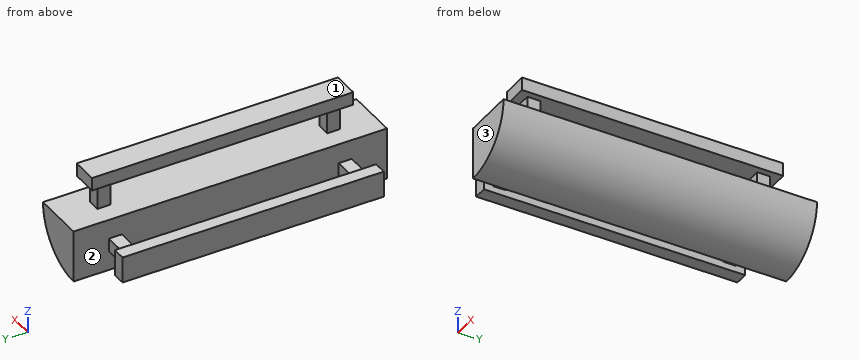
from build123d import *

# Parameters (mm, degrees)
SKETCH1_W               = 38.1
SKETCH1_H               = 101.6
BOSS_EXTRUDE1_DEPTH     = 304.8
CUT_EXTRUDE2_DEPTH      = 324.538575753
SKETCH3_W               = 12.7
SKETCH3_H               = 25.4
CUT_EXTRUDE3_DEPTH      = 324.538575753
CUT_EXTRUDE4_DEPTH      = 324.538575753
CUT_EXTRUDE5_DEPTH      = 152.4
SKETCH6_W               = 6.35
SKETCH6_H               = 6.35
BOSS_EXTRUDE2_DEPTH     = 12.7
SKETCH7_W               = 12.7
SKETCH7_H               = 127
BOSS_EXTRUDE3_DEPTH     = 6.35
MIRROR2_COPY_1_SKETCH_W = 6.35
MIRROR2_COPY_1_SKETCH_H = 6.35
MIRROR2_COPY_1_DEPTH    = 12.7


with BuildPart() as part:
    # Sketch1 → Boss-Extrude1 (new body)
    with BuildSketch(Plane(origin=(0, 0, 0), x_dir=(1, 0, 0), z_dir=(0, 1, 0))):
        with Locations((19.05, 50.8)):
            Rectangle(SKETCH1_W, SKETCH1_H)
    extrude(amount=BOSS_EXTRUDE1_DEPTH)

    # Sketch2 → Cut-Extrude2 (cut, through all)
    with BuildSketch(Plane.XZ):
        Polygon((12.7, -76.2), (38.1, -76.2), (38.1, 0), (0, 0), (0, -76.2), align=None)
    extrude(amount=-CUT_EXTRUDE2_DEPTH, mode=Mode.SUBTRACT)

    # Sketch3 → Cut-Extrude3 (cut, through all)
    with BuildSketch(Plane.XZ):
        with Locations((6.35, -88.9)):
            Rectangle(SKETCH3_W, SKETCH3_H)
    extrude(amount=-CUT_EXTRUDE3_DEPTH, mode=Mode.SUBTRACT)

    # Sketch4 → Cut-Extrude4 (cut, through all)
    with BuildSketch(Plane.XZ):
        with BuildLine():
            ThreePointArc((12.7, -101.6), (30.660512242, -94.160512242), (38.1, -76.2))
            Line((38.1, -76.2), (38.1, -101.6))
            Line((38.1, -101.6), (12.7, -101.6))
        make_face()
    extrude(amount=-CUT_EXTRUDE4_DEPTH, mode=Mode.SUBTRACT)

    # Sketch5 → Cut-Extrude5 (cut)
    with BuildSketch(Plane.XZ):
        with BuildLine():
            Line((12.7, -76.2), (12.7, -101.6))
            ThreePointArc((12.7, -101.6), (30.660512242, -94.160512242), (38.1, -76.2))
            Line((38.1, -76.2), (12.7, -76.2))
        make_face()
    extrude(amount=-CUT_EXTRUDE5_DEPTH, mode=Mode.SUBTRACT)

    # Sketch6 → Boss-Extrude2 (add)
    with BuildSketch(Plane.ZY.offset(-12.7)):
        with Locations((-88.9, 284.458069637)):
            Rectangle(SKETCH6_W, SKETCH6_H)
    boss_extrude2 = extrude(amount=BOSS_EXTRUDE2_DEPTH)

    # Mirror1: Boss-Extrude2 across plane
    add(boss_extrude2.mirror(Plane(origin=(0, 228.6, 0), x_dir=(0, 0, 1), z_dir=(0, -1, 0))))

    # Sketch7 → Boss-Extrude3 (add)
    with BuildSketch(Plane.ZY):
        with Locations((-88.9, 228.6)):
            Rectangle(SKETCH7_W, SKETCH7_H)
    boss_extrude3 = extrude(amount=BOSS_EXTRUDE3_DEPTH)

    # Mirror2: Boss-Extrude2, Boss-Extrude3 across plane
    add(boss_extrude2.mirror(Plane(origin=(-31.75, 0, -31.75), x_dir=(-0.7071067811865479, 0, 0.7071067811865471), z_dir=(0.7071067811865471, 0, 0.7071067811865479))))
    add(boss_extrude3.mirror(Plane(origin=(-31.75, 0, -31.75), x_dir=(-0.7071067811865479, 0, 0.7071067811865471), z_dir=(0.7071067811865471, 0, 0.7071067811865479))))

    # Mirror2 copy 1 sketch → Mirror2 copy 1 (add)
    with BuildSketch(Plane(origin=(-63.5, 457.2, -76.2), x_dir=(-1, 0, 0), z_dir=(0, 0, 1))):
        with Locations((-88.9, 284.458069637)):
            Rectangle(MIRROR2_COPY_1_SKETCH_W, MIRROR2_COPY_1_SKETCH_H)
    extrude(amount=MIRROR2_COPY_1_DEPTH)


solid = part.part
Can you work these out from the model? Positions are in its coordinate system, mm. Face numbers are marked on the shaded views. Round coordinates to 2 decimals unless told otherwise and drop trailing zeros. Loops run counter-clockwise (first coordinate to the right, second up) from the corner with the lowest first, then second, coordinate; pieces in that order, holes last. Notation, with made-up numbers: (79.25, 64) - (99.25, 64) arc R11 ccw to (99.25, 68) - close; hole circle Ø10 at (68.25, -14.5). An arc over 180 degrees is marked (long way). Use CSV: the item, a comma, the result in double quotes. Start each with the question number.
1) We'd pull the mould along Y, two halves only. Please class the marked faces 1, 2 and 3: released by +Y, released by -Y, zero draft, split by the parting line, or undercut.
2) If we section it at C-C on z = -90.5: Write out the boundary of the cut face in (x, y), plus the area to 3 significant figures.
3) For pin 1 Ø1.9 at (x, z) = (26, -59.5) entering from +Y; pin 2 Ø3 at (x, y) = (6.5, 173.5) entering from +Z (3 decimals); pin 3 Ø6.5 at (x, y) = (28.5, 229.5) entering from -Z, each with a flat end and sliding along its axis, tell me the tip position at first contact or that it passes through.
4) Please list where these lines run through material, in increasing order: probe 1 along Y at (x, z) = (5, -92); probe 2 along Z at (x, y) = (21, 246); probe 3 along X at (y, z) = (206, -86). Write a range as [from, to].
5) If we section it at A-A on x = 10.5: Write out the boundary of the cut face in (y, z) (3 decimals), plus the area to 3 significant figures.
6) If we section it at B-B on y = 168: Write out the boundary of the cut face in (x, z), plus the area to 3 significant figures.
7) If we section it at D-D on x = 26.5: Write out the boundary of the cut face in (y, z), plus the area to 3 significant figures.
Geometry results:
1,face 1,"zero draft"
1,face 2,"undercut"
1,face 3,"released by -Y"
2,outline,"(-6.35, 165.1) - (0, 165.1) - (0, 169.57) - (12.7, 169.57) - (12.7, 152.4) - (33.69, 152.4) - (33.69, 304.8) - (12.7, 304.8) - (12.7, 287.63) - (0, 287.63) - (0, 292.1) - (-6.35, 292.1) - close; hole (0, 175.92) - (12.7, 175.92) - (12.7, 281.28) - (0, 281.28) - close"
2,area,"4,170 mm2"
3,pin 1,"stops at y = 292.1"
3,pin 2,"stops at z = -85.725"
3,pin 3,"stops at z = -98.28"
4,probe 1,"y = [169.57, 175.92], [281.28, 287.63]"
4,probe 2,"z = [-100.21, -76.2], [-63.5, -57.15]"
4,probe 3,"x = [-6.35, 0], [12.7, 36.13]"
5,outline,"(169.567, -92.075) - (175.917, -92.075) - (175.917, -85.725) - (169.567, -85.725) - close; (281.283, -92.075) - (287.633, -92.075) - (287.633, -85.725) - (281.283, -85.725) - close"
5,area,"80.6 mm2"
6,outline,"(-6.35, -95.25) - (0, -95.25) - (0, -82.55) - (-6.35, -82.55) - close; (12.7, -101.6) arc R25.4 ccw to (38.1, -76.2) - (12.7, -76.2) - close; (19.05, -63.5) - (31.75, -63.5) - (31.75, -57.15) - (19.05, -57.15) - close"
6,area,"668 mm2"
7,outline,"(152.4, -97.52) - (304.8, -97.52) - (304.8, -76.2) - (287.63, -76.2) - (287.63, -63.5) - (292.1, -63.5) - (292.1, -57.15) - (165.1, -57.15) - (165.1, -63.5) - (169.57, -63.5) - (169.57, -76.2) - (152.4, -76.2) - close; hole (175.92, -76.2) - (281.28, -76.2) - (281.28, -63.5) - (175.92, -63.5) - close"
7,area,"4,220 mm2"
